from build123d import *

# Parameters (mm, degrees)
F1_DEPTH = 25.4


with BuildPart() as f1:
    # F0 (on Front) → F1 (new body)
    with BuildSketch(Plane.XZ):
        Polygon((-4.048808, 20.918848), (-53.984117, 20.918848), (-53.984117, -29.466329), (53.984117, -29.466329), (53.984117, 20.918848), (28.791532, 20.918848), align=None)
        with BuildLine():
            Line((-4.048808, 42.962365), (-4.048808, 20.918848))
            Line((-4.048808, 20.918848), (28.791532, 20.918848))
            Line((28.791532, 20.918848), (28.791532, 55.558659))
            ThreePointArc((28.791532, 55.558659), (53.670281, 86.397568), (89.073792, 68.604819))
            Line((89.073792, 68.604819), (89.073792, 77.152304))
            ThreePointArc((89.073792, 77.152304), (30.578157, 92.562694), (-4.048808, 42.962365))
        make_face()
        Polygon((89.073792, 96.946478), (89.073792, 77.152304), (89.073792, 68.604819), (89.073792, 57.358131), (162.852123, 57.358131), (162.852123, 96.946478), align=None)
    extrude(amount=F1_DEPTH)


solid = f1.part
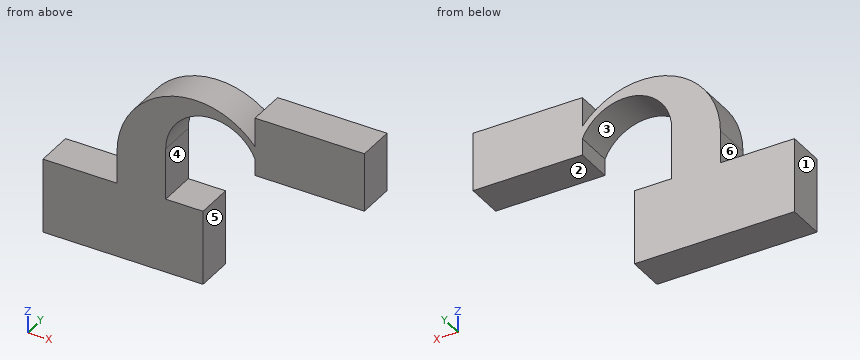
Work out the finished part from the listing and answer in its coordinate system (mm). Face numbers are marked on the shaded views. A direction names the side the tool comes from. Round coordinates to 2 decimals unless told otherwise and drop trailing zeros. Write each loop counter-clockwise with the first axis right and the second up, starting at its lowest first coordinate (ties: lowest second). Pieces come first, ordered by that corner, then holes. Notation, with made-up numbers: M -25,30 L 6,30 A16 ccw 6,53 Z; hole C -7,-10.5 d4. An arc over 180 degrees is marked long. Use a Markdown table: item, result.
1) The part is cut by section C-C on z = 64. Give the vertices of the cut face in (x, y), plus the area to 3 significant figures.
Taken from the geometry:
| item | result |
|---|---|
| outline | M 0.32,-25.4 L 29.94,-25.4 L 29.94,0 L 0.32,0 Z; M 89.07,-25.4 L 162.85,-25.4 L 162.85,0 L 89.07,0 Z |
| area | 2,630 mm2 |
2) Which of the six approach directions +Z, -Z, +X, -X, +Y, -Y give full straight-line access (tool end or side, diameter ignored) to the marked faces 4, 5 and 6?
Taken from the geometry:
| item | result |
|---|---|
| face 4 | +X, +Y, -Y |
| face 5 | -Z, +X, +Y, -Y |
| face 6 | +Z, -X, +Y, -Y |
3) The part is cut by section B-B on x = 44. Give the vertices of the cut face in (y, z).
Taken from the geometry:
| item | result |
|---|---|
| outline | M -25.4,-29.47 L 0,-29.47 L 0,20.92 L -25.4,20.92 Z; M -25.4,82.55 L 0,82.55 L 0,95.58 L -25.4,95.58 Z |
4) Consider line 1 (Z direction, x = 121.5, y = -2.5); line 2 (X direction, y = -10.5, z = -4); line 3 (X direction, y = -8.25, z = 22). Determine where each line is inside the solid, lowest interval first. Write a range as [from, to].
Taken from the geometry:
| item | result |
|---|---|
| line 1 | z = [57.36, 96.95] |
| line 2 | x = [-53.98, 53.98] |
| line 3 | x = [-4.05, 28.79] |
5) Flat-ended cylindrical pins translate along their axes: pin 1 (12.5 mm diameter, centred on x = 121, y = -15, fed in from -Z); pin 2 (1.5 mm diameter, centred on x = 57, y = -21.5, fed in from -Z); pin 3 (7.5 mm diameter, centred on y = -12, z = 39.5, fed in from +X). Find the tip coordinate at first contact, or state that the pin passes through.
Taken from the geometry:
| item | result |
|---|---|
| pin 1 | stops at z = 57.36 |
| pin 2 | stops at z = 86.84 |
| pin 3 | stops at x = 28.79 |
6) Determine the mould class of the marked faces 1, 2 and 3 for opening direction Z: pulls with the +Z half, pulls with the -Z half, needs draft (parallel to the pull), parting line crosses it, or undercut.
Taken from the geometry:
| item | result |
|---|---|
| face 1 | needs draft |
| face 2 | pulls with the -Z half |
| face 3 | undercut |
7) The part is cut by section A-A on y = -13.75. Give the vertices of the cut face in (x, z).
Taken from the geometry:
| item | result |
|---|---|
| outline | M -53.98,-29.47 L 53.98,-29.47 L 53.98,20.92 L 28.79,20.92 L 28.79,55.56 A31.55 cw 89.07,68.6 L 89.07,57.36 L 162.85,57.36 L 162.85,96.95 L 89.07,96.95 L 89.07,77.15 A52.84 ccw -4.05,42.96 L -4.05,20.92 L -53.98,20.92 Z |
8) The part is cut by section D-D on x = 111. Give the vertices of the cut face in (y, z).
Taken from the geometry:
| item | result |
|---|---|
| outline | M -25.4,57.36 L 0,57.36 L 0,96.95 L -25.4,96.95 Z |
